The drawing under review shows one solid part. Ordinate dimensions are in mm from its lowest x, y, z. A direction names the side the tool comes from. Give positions to 0.01 mm unless a question says otherwise; leave off trailing zeros. Loops run counter-clockwise (first coordinate to the right, second up) from the corner with the lowest first, then second, coordinate; pieces in that order, holes last. Notation, with made-up numbers: (-9.75, 24.5) -> (22.25, 24.5) arc R12 ccw to (22.25, 43.5) -> close; hole circle Ø11 at (35.5, 63). An arc over 180 degrees is marked (long way). Answer in a Markdown table with one row per item. Add a question column.
(1) Consider section D-D on z = 18. Write out the cut boundary in (x, y) (3 decimals), then the cut area to 3 significant figures.
(2) Consider section B-B on x = 105. Write out the cut boundary in (y, z) (3 decimals), then the cut area to 3 significant figures.
(3) Draft analysis for pull direction X (two halves, no side actions). For the marked faces 1, 2 and 3, state which applies: +X half, -X half, draft (parallel to the pull), parting line (faces both ways), or undercut.
(4) Consider section C-C on y = 19.5. Write out the cut boundary in (x, z).
(5) For the marked faces 4 and 5, list the 3-axis set-ups (+Z, -Z, +X, -X, +Y, -Y) from which the entire face can be reached by the end or side of a thin tool; tool diameter is ignored.
(6) For line 1 (Y direction, x = 80, z = 38.1); line 2 (Z direction, x = 34, y = 19.5); line 3 (X direction, y = 26.5, z = 11), list the stretches that pass through material, from the lowest coordinate up.
(7) Consider section A-A on z = 43.5. Write out the cut boundary in (x, y) (3 decimals).
(8) For pin 1 (7.5 mm diameter, centred on y = 26, z = 32, fed in from -X), flat-tipped, find the tip position at first contact; note if it passes through.
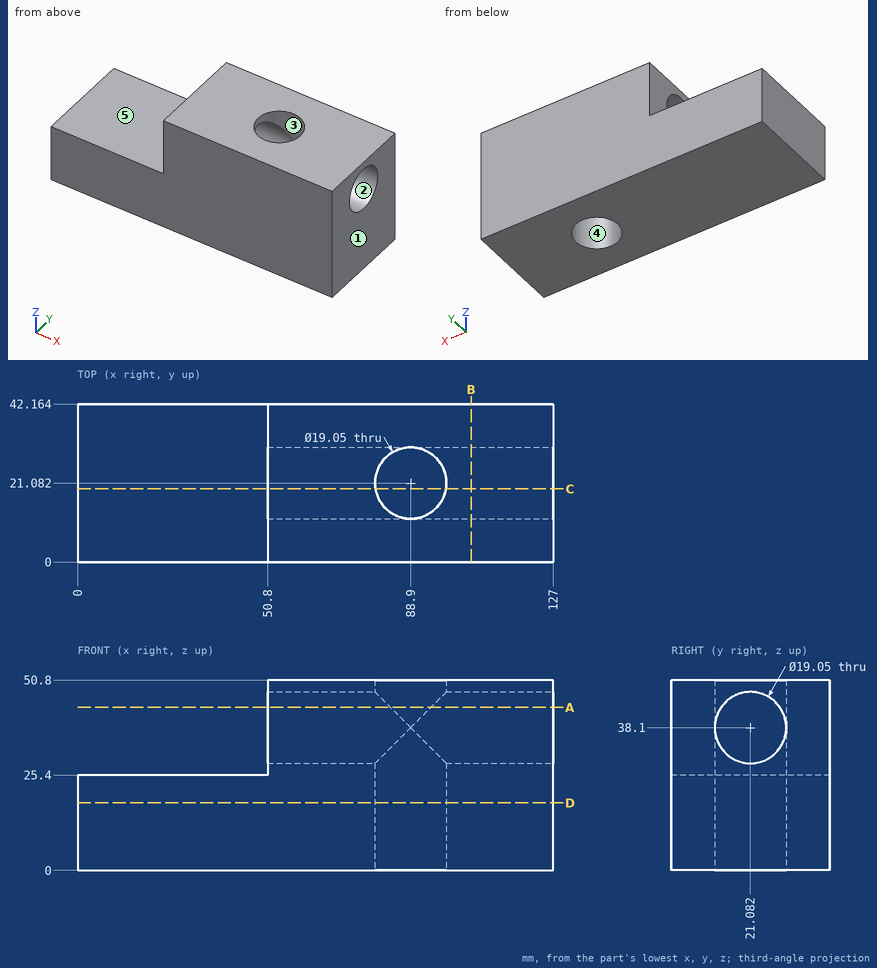
Values follow:
| question | item | result |
|---|---|---|
| 1 | outline | (0, 0) -> (127, 0) -> (127, 42.164) -> (0, 42.164) -> close; hole circle Ø19.05 at (88.9, 21.082) |
| 1 | area | 5,070 mm2 |
| 2 | outline | (0, 0) -> (42.164, 0) -> (42.164, 50.8) -> (0, 50.8) -> close; hole circle Ø19.05 at (21.082, 38.1) |
| 2 | area | 1,860 mm2 |
| 3 | face 1 | +X half |
| 3 | face 2 | draft |
| 3 | face 3 | undercut |
| 4 | outline | (0, 0) -> (79.51, 0) -> (79.51, 28.71) -> (50.8, 28.71) -> (50.8, 25.4) -> (0, 25.4) -> close; (50.8, 47.49) -> (79.51, 47.49) -> (79.51, 50.8) -> (50.8, 50.8) -> close; (98.29, 0) -> (127, 0) -> (127, 28.71) -> (98.29, 28.71) -> close; (98.29, 47.49) -> (127, 47.49) -> (127, 50.8) -> (98.29, 50.8) -> close |
| 5 | face 4 | +Z, -Z |
| 5 | face 5 | +Z, -X, +Y, -Y |
| 6 | line 1 | 0 to 11.56, 30.61 to 42.16 |
| 6 | line 2 | 0 to 25.4 |
| 6 | line 3 | 0 to 81.07, 96.73 to 127 |
| 7 | outline | (50.8, 0) -> (127, 0) -> (127, 13.236) -> (94.3, 13.236) arc R9.525 cw to (83.5, 13.236) -> (50.8, 13.236) -> close; (50.8, 28.928) -> (83.5, 28.928) arc R9.525 cw to (94.3, 28.928) -> (127, 28.928) -> (127, 42.164) -> (50.8, 42.164) -> close |
| 8 | pin 1 | x = 50.8 |
